Geometry check sheet. Reference: the model listing, model coordinates, mm. Face numbers are marked on the shaded views. A direction names the side the tool comes from. Round coordinates to 2 decimals unless told otherwise and drop trailing zeros. Order: outer loops, then holes, each group sorted by start corner. A loop starts at its lowest first (then second) coordinate and runs counter-clockwise, first axis right, second up. Notation, with made-up numbers: (-40, 12) - (-7, 12) arc R29 cw to (-7, 34) - close; hole circle Ø7 at (55.5, -6.5). An arc over 180 degrees is marked (long way). One line per question, with ' | ' between items. Start each with the question number.
Q1. Mould release check, pull along X, two halves, no side actions. Record for the marked faces 3 and 4: +X half, -X half, draft (parallel to the pull), parting line (faces both ways), or undercut.
Q2. Sectioned sample at B-B, the plane y = 9.5. Enter the section's corners in (x, z).
Q3. Tool access check on the marked faces 1 and 2. Record the directions out of +Z, -Z, +X, -X, +Y, -Y that give a thin tool (end or side, any length) a straight path to the whole face; none if there is none.
Q4. Sectioned sample at A-A, the plane z = 39.5. Enter the section's corners in (x, y) (3 decimals), then the cut area to 3 significant figures.
Q5. Sectioned sample at C-C, the plane z = 12. Enter the section's corners in (x, y).
Q6. Material ranges on line 1 along Y through (x, z) = (7, 157); line 2 along Z through (x, y) = (27.5, 2.75); line 3 along X through (y, z) = (18.75, 87), recorded low to high.
Q7. Sectioned sample at D-D, the plane x = 8.5. Enter the section's corners in (y, z).
Q8. Gauge pin test, flat ends, axial feed: P1, Ø10, axis at y = 16.5, z = 112.5, coming from the -X side; P2, Ø12, axis at y = 15, z = 81, coming from the -X side; P3, Ø7, axis at x = 31.5, y = 2, coming from the -Z side; P4, Ø4.5, axis at x = 30.6, y = 2.38, coming from the +Z side. Record the tip position at first contact, or that the pin passes through.
```python
from build123d import *

# Parameters (mm, degrees)
BOSS_EXTRUDE1_OUTLINE_R = 2.54
BOSS_EXTRUDE1_DEPTH     = 184.2
CUT_EXTRUDE4_START      = -22.098
CUT_EXTRUDE4_DEPTH      = 22.098
CUT_EXTRUDE5_DEPTH      = 22.098


# Read off the part's stored shape, not the designer's step: Boss-Extrude1
with BuildPart() as part:
    # Boss-Extrude1 outline → Boss-Extrude1 (new body)
    with BuildSketch(Plane.XY):
        with BuildLine():
            Line((25, 0), (26.841758653, 0))
            ThreePointArc((26.841758653, 0), (34.864700777, 3.619120343), (26.150906359, 2.38))
            Line((26.150906359, 2.38), (25.625906359, 2.38))
            Line((25.625906359, 2.38), (13.5, 23.382685902))
            Line((13.5, 23.382685902), (-13.5, 23.382685902))
            Line((-13.5, 23.382685902), (-27, 0))
            Line((-27, 0), (-25, 0))
            Line((-25, 0), (-12.5, 21.650635095))
            Line((-12.5, 21.650635095), (12.5, 21.650635095))
            Line((12.5, 21.650635095), (25, 0))
        make_face()
        with Locations((30.595906359, 2.38)):
            Circle(BOSS_EXTRUDE1_OUTLINE_R, mode=Mode.SUBTRACT)
    extrude(amount=BOSS_EXTRUDE1_DEPTH)

    # Sketch5 → Cut-Extrude4 (cut)
    with BuildSketch(Plane.XY.offset(184.2).offset(CUT_EXTRUDE4_START)):
        with BuildLine():
            Line((23.625906359, 2.38), (26.150906359, 2.38))
            ThreePointArc((26.150906359, 2.38), (34.864700777, 3.619120342), (26.841758653, 0))
            Line((26.841758653, 0), (25, 0))
            Line((25, 0), (23.625906359, 2.38))
        make_face()
    extrude(amount=CUT_EXTRUDE4_DEPTH, mode=Mode.SUBTRACT)

    # Sketch6 → Cut-Extrude5 (cut)
    with BuildSketch(Plane(origin=(0, 0, 0), x_dir=(-1, 0, 0), z_dir=(0, 0, -1))):
        with BuildLine():
            Line((-23.625906359, 2.38), (-26.150906359, 2.38))
            ThreePointArc((-26.150906359, 2.38), (-34.864700777, 3.619120342), (-26.841758653, 0))
            Line((-26.841758653, 0), (-25, 0))
            Line((-25, 0), (-23.625906359, 2.38))
        make_face()
    extrude(amount=-CUT_EXTRUDE5_DEPTH, mode=Mode.SUBTRACT)


solid = part.part
```
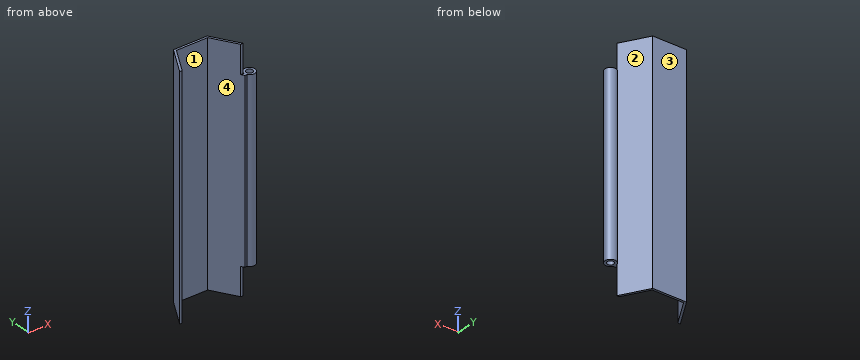
Determined:
1) face 3: draft | face 4: undercut
2) outline: (-21.52, 0) - (-19.52, 0) - (-19.52, 184.2) - (-21.52, 184.2) - close; (19.52, 0) - (21.52, 0) - (21.52, 184.2) - (19.52, 184.2) - close
3) face 1: +Z, -Z, -Y | face 2: +Z, -Z, +Y
4) outline: (-27, 0) - (-25, 0) - (-12.5, 21.651) - (12.5, 21.651) - (25, 0) - (26.842, 0) arc R4.445 ccw (long way) to (26.151, 2.38) - (25.626, 2.38) - (13.5, 23.383) - (-13.5, 23.383) - close; hole circle Ø5.08 at (30.596, 2.38) | area: 177 mm2
5) outline: (-27, 0) - (-25, 0) - (-12.5, 21.65) - (12.5, 21.65) - (23.63, 2.38) - (25.63, 2.38) - (13.5, 23.38) - (-13.5, 23.38) - close
6) line 1: y = 21.65 to 23.38 | line 2: z = 22.1 to 162.1 | line 3: x = -16.17 to -14.17, 14.17 to 16.17
7) outline: (21.65, 0) - (23.38, 0) - (23.38, 184.2) - (21.65, 184.2) - close
8) P1: stops at x = -20.36 | P2: stops at x = -21.8 | P3: stops at z = 22.1 | P4: passes through
